Check sheet for the drawn part. Datum: minimum x, y, z corner. Units: mm. A direction names the side the tool comes from. Give positions to 0.01 mm unless a question says otherwise; leave off trailing zeros. Write each loop counter-clockwise with the first axis right and the second up, starting at its lowest first coordinate (ties: lowest second). Pieces come first, ordered by that corner, then holes. Notation, with made-up numbers: (-28.5, 65.5) -> (0.5, 65.5) arc R13 cw to (0.5, 82.5) -> close; hole circle Ø7 at (53, -40). An arc over 180 degrees is marked (long way). Use CSV: the item, a comma, the result in double quotes. Start each with the question number.
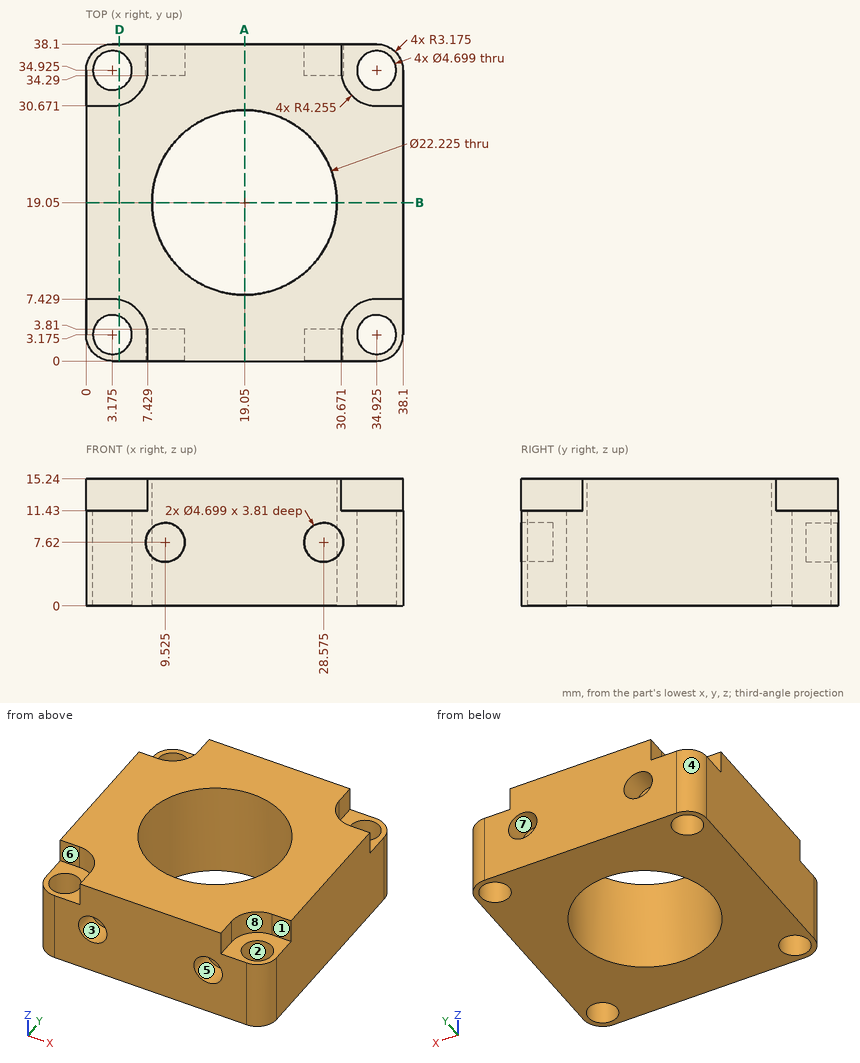
(1) Set-up check for the marked faces 4, 5, 6, 7 and 8: record each of +Z, -Z, +X, -X, +Y, -Y from which the full face is reachable in a straight line by a thin tool's end or side.
(2) Thickness scan on line 1 (X direction, y = 35, z = 10.25); line 2 (Z direction, x = 28.5, y = 2.5); line 3 (X direction, y = 36.7, z = 7.62) (1 decimal). Record the ranges inside material, lowest first. Write a range as from..to.
(3) Draft check along Y on the marked faces 1, 2 and 3. Enter one of: released by +Y, released by -Y, zero draft, split by the parting line, or undercut.
(4) Section check A-A on x = 19.05. Record the cut outline in (y, z).
(5) Go/stop test with flat-tipped pins: pin 1 (4 mm diameter, centred on x = 3.175, y = 34.925, fed in from +Z); pin 2 (3 mm diameter, centred on y = 28, z = 7, fed in from -X); pin 3 (3.5 mm diameter, centred on x = 3, y = 5, fed in from +Z); pin 4 (1.6 mm diameter, centred on y = 1, z = 14, fed in from +X). Record where each tip stops, or that it passes through.
(6) Section check D-D on x = 4. Record the cut outline in (y, z) (1 decimal), then the cut area to 3 significant figures.
Data:
1,face 4,"+Z, -Z, -X, +Y"
1,face 5,"-Y"
1,face 6,"+Z, -X, -Y"
1,face 7,"+Y"
1,face 8,"+Z, +X, -Y"
2,line 1,"x = 0..0.83, 5.52..32.58, 37.27..38.1"
2,line 2,"z = 0..5.27, 9.97..15.24"
2,line 3,"x = 0.5..1.6, 4.7..7.2, 11.9..26.2, 30.9..33.4, 36.5..37.6"
3,face 1,"released by -Y"
3,face 2,"undercut"
3,face 3,"zero draft"
4,outline,"(0, 0) -> (7.94, 0) -> (7.94, 15.24) -> (0, 15.24) -> close; (30.16, 0) -> (38.1, 0) -> (38.1, 15.24) -> (30.16, 15.24) -> close"
5,pin 1,"passes through"
5,pin 2,"stops at x = 0"
5,pin 3,"stops at z = 11.43"
5,pin 4,"stops at x = 30.67"
6,outline,"(0, 0) -> (1, 0) -> (1, 11.4) -> (0, 11.4) -> close; (5.4, 0) -> (32.7, 0) -> (32.7, 11.4) -> (30.8, 11.4) -> (30.8, 15.2) -> (7.3, 15.2) -> (7.3, 11.4) -> (5.4, 11.4) -> close; (37.1, 0) -> (38.1, 0) -> (38.1, 11.4) -> (37.1, 11.4) -> close"
6,area,"424 mm2"
